Source: CAD feature listing. Evaluate the final solid. Frame: model axes, mm. A direction names the side the tool comes from. Round coordinates to 2 decimals unless told otherwise and drop trailing zeros. Order: outer loops, then holes, each group sorted by start corner. A loop starts at its lowest first (then second) coordinate and runs counter-clockwise, first axis right, second up. Notation, with made-up numbers: M -34,-1.75 L 2,-1.75 A17 ccw 2,2.25 Z; hole C 29,70.25 d3. An arc over 180 degrees is marked long. Use one line per item in the form item = value. Start each with the question number.
Q1. Section C-C (y = 1). Return the cut outline in (x, z).
Q2. Contact query for flat-ended pins moving along their axis: pin 1 (4 mm diameter, centred on y = 5, z = 1, fed in from +X); pin 2 (12 mm diameter, centred on x = -14, y = -7, fed in from -Z); pin 3 (1.5 mm diameter, centred on y = 4, z = -3, fed in from -X). Output: stop coordinate, or through.
Q3. Reachability of faces 4 (the flat face through (-5, 0, -3)), 5 (the flat face through (5, 0, -3)), 6 (the cylindrical face through (6.225, -2.956, -2.535)), 7 (the flat face through (-3.067, -3.501, -2.571)), 8 (the cylindrical face through (18.82, 1.08, 1.97)) from +Z, -Z, +X, -X, +Y, -Y: full face, straight path, thin tool, end or side. Return the list, or none.
Q4. Section B-B (z = 0.75). Return the cut outline in (x, y).
Q5. Pull-direction query (X, two-part tool) for faces 1 (the flat face through (0, 0, 4)), 2 (the cylindrical face through (-12.462, 4.275, 1.972)), 3 (the cylindrical face through (-6.2, -3.01, -2.54)); classes: pulls with the +X half, pulls with the -X half, needs draft (parallel to the pull), parting line crosses it, or undercut.
Q6. Section D-D (z = -5.75). Return the cut outline in (x, y), plus the area to 3 significant figures.
Q7. Section A-A (x = -20). Return the cut outline in (y, z).
Q8. Material intervals for probe 1 along Y at (x, z) = (20, 1.55); probe 2 along Z at (x, y) = (19, 3.75); probe 3 along Y at (x, z) = (0, -0.25), sorted ascending.
from build123d import *

# Parameters (mm, degrees)
CORTE_EXTRUS_O1_DEPTH    = 12.838758968
ESBO_O4_R                = 1.6
RESSALTO_EXTRUS_O1_DEPTH = 4


with BuildPart() as part:
    # Esboço1 → Revolução1 (revolve)
    with BuildSketch(Plane(origin=(0, 0, 0), x_dir=(1, 0, 0), z_dir=(0, 1, 0))):
        with BuildLine():
            Line((0, 0), (6.891534421, 0))
            Line((6.891534421, 0), (6.891534421, 5))
            ThreePointArc((6.891534421, 5), (6.180613943, 6.309516298), (4.743586175, 6.703460527))
            ThreePointArc((4.743586175, 6.703460527), (3.710745118, 2.736851933), (0, 0.995842151))
            Line((0, 0.995842151), (0, 0))
        make_face()
    revolve(axis=Axis((0, 0, 0), (0, 0, -1)))

    # Esboço3 → Corte-extrusão1 (cut, through all)
    with BuildSketch(Plane.XY):
        with BuildLine():
            Line((-2, 19.326317369), (-2, 1.734101615))
            Line((-2, 1.734101615), (-17.937282026, -7.467292453))
            ThreePointArc((-17.937282026, -7.467292453), (-16.698748021, 9.932691356), (-2, 19.326317369))
        make_face()
        with BuildLine():
            Line((2, 19.326317369), (2, 1.734101615))
            Line((2, 1.734101615), (17.937282026, -7.467292453))
            ThreePointArc((17.937282026, -7.467292453), (16.698748021, 9.932691356), (2, 19.326317369))
        make_face()
        with BuildLine():
            Line((0, -1.73), (-16.027252382, -10.983338477))
            ThreePointArc((-16.027252382, -10.983338477), (0, -19.429527607), (16.027252382, -10.983338477))
            Line((16.027252382, -10.983338477), (0, -1.73))
        make_face()
    extrude(amount=-CORTE_EXTRUS_O1_DEPTH, mode=Mode.SUBTRACT)

    # Esboço4 → Ressalto-extrusão1 (add)
    with BuildSketch(Plane.XY):
        with BuildLine():
            ThreePointArc((-6.64, -7.477325725), (0, -10), (6.64, -7.477325725))
            ThreePointArc((6.64, -7.477325725), (12.553949294, -4.249302623), (19.284210526, -3.935434592))
            ThreePointArc((19.284210526, -3.935434592), (24, 0), (19.284210526, 3.935434592))
            ThreePointArc((19.284210526, 3.935434592), (12.553949294, 4.249302623), (6.64, 7.477325725))
            ThreePointArc((6.64, 7.477325725), (0, 10), (-6.64, 7.477325725))
            ThreePointArc((-6.64, 7.477325725), (-12.553949294, 4.249302623), (-19.284210526, 3.935434592))
            ThreePointArc((-19.284210526, 3.935434592), (-24, 0), (-19.284210526, -3.935434592))
            ThreePointArc((-19.284210526, -3.935434592), (-12.553949294, -4.249302623), (-6.64, -7.477325725))
        make_face()
        with Locations((20, 0)):
            Circle(ESBO_O4_R, mode=Mode.SUBTRACT)
        with Locations((-20, 0)):
            Circle(ESBO_O4_R, mode=Mode.SUBTRACT)
    extrude(amount=RESSALTO_EXTRUS_O1_DEPTH)


solid = part.part
Results list:
q1.outline = M -23.87,0 L -21.25,0 L -21.25,4 L -23.87,4 Z; M -18.75,0 L -3.27,0 L -3.27,-2.42 A4.72 cw 3.27,-2.42 L 3.27,0 L 18.75,0 L 18.75,4 L -18.75,4 Z; M 21.25,0 L 23.87,0 L 23.87,4 L 21.25,4 Z
q2.pin_1 = 22.65
q2.pin_2 = 0
q2.pin_3 = -2
q3.face_4 = -Z, -X, +Y
q3.face_5 = -Z, +X, +Y
q3.face_6 = -Z, +X, -Y
q3.face_7 = -Z, -Y
q3.face_8 = +Z, -Z
q4.outline = M -19.28,-3.94 A15 cw -6.64,-7.48 A10 ccw 6.64,-7.48 A15 cw 19.28,-3.94 A4 ccw long 19.28,3.94 A15 cw 6.64,7.48 A10 ccw -6.64,7.48 A15 cw -19.28,3.94 A4 ccw long Z; hole C -20,0 d3.2; hole C 20,0 d3.2
q5.face_1 = needs draft
q5.face_2 = undercut
q5.face_3 = pulls with the -X half
q6.outline = M -6.59,-0.92 A6.66 ccw -4.87,-4.54 L -3.22,-3.59 A4.82 cw -4.82,0.1 Z; M -2,4.39 A4.82 cw 2,4.39 L 2,6.35 A6.66 ccw -2,6.35 Z; M 3.22,-3.59 L 4.87,-4.54 A6.66 ccw 6.59,-0.92 L 4.82,0.1 A4.82 cw Z
q6.area = 22.6 mm2
q7.outline = M -4,0 L -1.6,0 L -1.6,4 L -4,4 Z; M 1.6,0 L 4,0 L 4,4 L 1.6,4 Z
q8.probe_1 = -4 to -1.6, 1.6 to 4
q8.probe_2 = 0 to 4
q8.probe_3 = -1.73 to 6.89
